Could you check a few things on this model? Use its own coordinates, in mm. Face numbers are marked on the shaded views. A direction names the side the tool comes from. Give positions to 0.01 mm unless a question says otherwise; leave off trailing zeros. Write each loop counter-clockwise with the first axis right and the second up, starting at its lowest first coordinate (ties: lowest second). Pieces come first, ordered by that corner, then holes. Notation, with made-up numbers: M 44.25,41.5 L 78.25,41.5 A15 ccw 78.25,68.5 Z; hole C 50.5,38 d11. An arc over 180 degrees is marked long. Use one line per item in the form item = value.
from build123d import *

# Parameters (mm, degrees)
SKETCH7_W           = 32.8
SKETCH7_H           = 24.5
BOSS_EXTRUDE3_DEPTH = 19
SKETCH8_W           = 29.8
SKETCH8_H           = 24.5
BOSS_EXTRUDE4_DEPTH = 7
CUT_EXTRUDE1_DEPTH  = 23.5
CUT_EXTRUDE2_REACH  = 44.494
SKETCH10_W          = 2.7
SKETCH10_H          = 21.05
SKETCH18_W          = 3
SKETCH18_H          = 8
CUT_EXTRUDE3_DEPTH  = 1
CHAMFER1_SIZE       = 0.5
CUT_EXTRUDE5_REACH  = 44.494
SKETCH20_R          = 0.6
CUT_EXTRUDE6_REACH  = 44.494
SKETCH19_R          = 0.6
CUT_EXTRUDE7_REACH  = 35.091
SKETCH21_R          = 2.25
SKETCH21_R_2        = 1.25
CHAMFER2_SIZE       = 0.5
CHAMFER4_SIZE       = 0.2


with BuildPart() as part:
    # Sketch7 → Boss-Extrude3 (new body)
    with BuildSketch(Plane.XY):
        Rectangle(SKETCH7_W, SKETCH7_H)
    extrude(amount=BOSS_EXTRUDE3_DEPTH)

    # Sketch8 → Boss-Extrude4 (add)
    with BuildSketch(Plane.XY.offset(19)):
        Rectangle(SKETCH8_W, SKETCH8_H)
    extrude(amount=BOSS_EXTRUDE4_DEPTH)

    # Sketch16 → Cut-Extrude1 (cut)
    with BuildSketch(Plane.XY.offset(26)):
        with BuildLine():
            Line((-12.4, -11.25), (12.4, -11.25))
            ThreePointArc((12.4, -11.25), (13.460660172, -10.810660172), (13.9, -9.75))
            Line((13.9, -9.75), (13.9, 9.75))
            ThreePointArc((13.9, 9.75), (13.460660172, 10.810660172), (12.4, 11.25))
            Line((12.4, 11.25), (-12.4, 11.25))
            ThreePointArc((-12.4, 11.25), (-13.460660172, 10.810660172), (-13.9, 9.75))
            Line((-13.9, 9.75), (-13.9, -9.75))
            ThreePointArc((-13.9, -9.75), (-13.460660172, -10.810660172), (-12.4, -11.25))
        make_face()
    extrude(amount=-CUT_EXTRUDE1_DEPTH, mode=Mode.SUBTRACT)

    # Cut-Extrude2: up to this face of the body (flat: up to its plane)
    cut_extrude2_end = Plane(part.part.faces().sort_by_distance((14.9, 0, 22.5))[0])
    # Sketch10 → Cut-Extrude2 (cut, up to the picked face)
    with BuildSketch(Plane.ZY.offset(14.9), mode=Mode.PRIVATE) as cut_extrude2_sk1:
        with Locations((24.65, 0.725)):
            Rectangle(SKETCH10_W, SKETCH10_H)
    cut_extrude2_tool1 = split(extrude(cut_extrude2_sk1.sketch, amount=-CUT_EXTRUDE2_REACH, mode=Mode.PRIVATE), bisect_by=cut_extrude2_end, keep=Keep.BOTH, mode=Mode.PRIVATE)
    add(cut_extrude2_tool1.solids().sort_by(Axis((-14.9, 0.725, 24.65), (1, 0, 0)))[0], mode=Mode.SUBTRACT)

    # Sketch18 → Cut-Extrude3 (cut)
    with BuildSketch(Plane(origin=(14.9, 0, 0), x_dir=(0, 0, -1), z_dir=(1, 0, 0))):
        with Locations((-21.8, 3.95)):
            Rectangle(SKETCH18_W, SKETCH18_H)
    extrude(amount=-CUT_EXTRUDE3_DEPTH, mode=Mode.SUBTRACT)

    # Chamfer1
    chamfer1_edges = [part.edges().sort_by_distance(p)[0] for p in [
        (0, -12.25, 0),
        (-16.4, 0, 0),
        (0, 12.25, 0),
        (16.4, 0, 0),
        (16.4, -12.25, 9.5),
        (-16.4, -12.25, 9.5),
        (-16.4, 12.25, 9.5),
        (16.4, 12.25, 9.5),
    ]]
    chamfer(chamfer1_edges, length=CHAMFER1_SIZE)

    # Sketch20 → Cut-Extrude5 (cut, up to next)
    with BuildSketch(Plane(origin=(14.9, 0, 0), x_dir=(0, 0, -1), z_dir=(1, 0, 0)), mode=Mode.PRIVATE) as cut_extrude5_sk1:
        with Locations((-21.5, 10)):
            Circle(SKETCH20_R)
    cut_extrude5_tool1 = extrude(cut_extrude5_sk1.sketch, amount=-CUT_EXTRUDE5_REACH, mode=Mode.PRIVATE) & part.part
    # Sketch20 → Cut-Extrude5 (cut, up to next)
    with BuildSketch(Plane(origin=(14.9, 0, 0), x_dir=(0, 0, -1), z_dir=(1, 0, 0)), mode=Mode.PRIVATE) as cut_extrude5_sk2:
        with Locations((-21.5, -10)):
            Circle(SKETCH20_R)
    cut_extrude5_tool2 = extrude(cut_extrude5_sk2.sketch, amount=-CUT_EXTRUDE5_REACH, mode=Mode.PRIVATE) & part.part
    add(cut_extrude5_tool1.solids().sort_by_distance((14.9, 10, 21.5))[0], mode=Mode.SUBTRACT)
    add(cut_extrude5_tool2.solids().sort_by_distance((14.9, -10, 21.5))[0], mode=Mode.SUBTRACT)

    # Sketch19 → Cut-Extrude6 (cut, up to next)
    with BuildSketch(Plane.ZY.offset(14.9), mode=Mode.PRIVATE) as cut_extrude6_sk1:
        with Locations(Location((21.5, 10, 0), (0, 0, 180))):
            Circle(SKETCH19_R)
    cut_extrude6_tool1 = extrude(cut_extrude6_sk1.sketch, amount=-CUT_EXTRUDE6_REACH, mode=Mode.PRIVATE) & part.part
    # Sketch19 → Cut-Extrude6 (cut, up to next)
    with BuildSketch(Plane.ZY.offset(14.9), mode=Mode.PRIVATE) as cut_extrude6_sk2:
        with Locations(Location((21.5, -10, 0), (0, 0, 180))):
            Circle(SKETCH19_R)
    cut_extrude6_tool2 = extrude(cut_extrude6_sk2.sketch, amount=-CUT_EXTRUDE6_REACH, mode=Mode.PRIVATE) & part.part
    add(cut_extrude6_tool1.solids().sort_by_distance((-14.9, 10, 21.5))[0], mode=Mode.SUBTRACT)
    add(cut_extrude6_tool2.solids().sort_by_distance((-14.9, -10, 21.5))[0], mode=Mode.SUBTRACT)

    # Sketch21 → Cut-Extrude7 (cut, up to next)
    with BuildSketch(Plane(origin=(0, 0, 0), x_dir=(-1, 0, 0), z_dir=(0, 0, -1)), mode=Mode.PRIVATE) as cut_extrude7_sk1:
        with Locations((-10.65, 0)):
            Circle(SKETCH21_R)
    cut_extrude7_tool1 = extrude(cut_extrude7_sk1.sketch, amount=-CUT_EXTRUDE7_REACH, mode=Mode.PRIVATE) & part.part
    # Sketch21 → Cut-Extrude7 (cut, up to next)
    with BuildSketch(Plane(origin=(0, 0, 0), x_dir=(-1, 0, 0), z_dir=(0, 0, -1)), mode=Mode.PRIVATE) as cut_extrude7_sk2:
        with Locations((0, 6)):
            Circle(SKETCH21_R_2)
    cut_extrude7_tool2 = extrude(cut_extrude7_sk2.sketch, amount=-CUT_EXTRUDE7_REACH, mode=Mode.PRIVATE) & part.part
    # Sketch21 → Cut-Extrude7 (cut, up to next)
    with BuildSketch(Plane(origin=(0, 0, 0), x_dir=(-1, 0, 0), z_dir=(0, 0, -1)), mode=Mode.PRIVATE) as cut_extrude7_sk3:
        with Locations((0, -6)):
            Circle(SKETCH21_R_2)
    cut_extrude7_tool3 = extrude(cut_extrude7_sk3.sketch, amount=-CUT_EXTRUDE7_REACH, mode=Mode.PRIVATE) & part.part
    add(cut_extrude7_tool1.solids().sort_by_distance((10.65, 0, 0))[0], mode=Mode.SUBTRACT)
    add(cut_extrude7_tool2.solids().sort_by_distance((0, 6, 0))[0], mode=Mode.SUBTRACT)
    add(cut_extrude7_tool3.solids().sort_by_distance((0, -6, 0))[0], mode=Mode.SUBTRACT)

    # Chamfer2
    chamfer2_edges = [part.edges().sort_by_distance(p)[0] for p in [
        (12.9, 0, 0),
    ]]
    chamfer(chamfer2_edges, length=CHAMFER2_SIZE)

    # Chamfer4
    chamfer4_edges = [part.edges().sort_by_distance(p)[0] for p in [
        (1.25, 6, 2.5),
        (1.25, 6, 0),
        (1.25, -6, 2.5),
        (1.25, -6, 0),
        (12.9, 0, 2.5),
    ]]
    chamfer(chamfer4_edges, length=CHAMFER4_SIZE)


solid = part.part
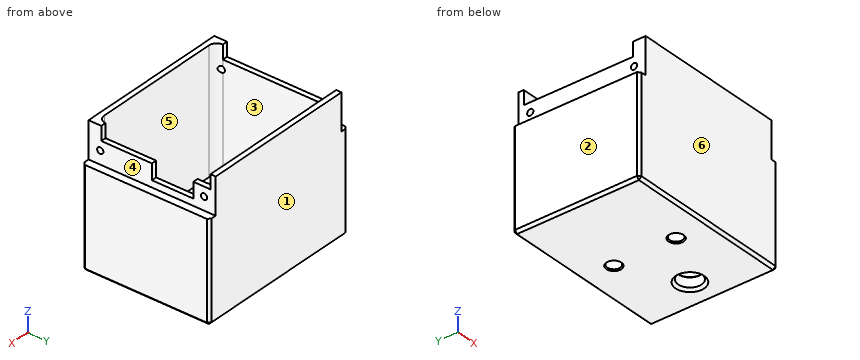
1) Thinking about a two-plate mould opening in Y: for the marked faces 1, 2 and 3, which applies, released by +Y, released by -Y, zero draft, split by the parting line, or undercut?
Checked values:
face_1 = released by +Y
face_2 = zero draft
face_3 = undercut
2) I want a section at B-B, the plane y = 6. Please give me the cut outline in (x, z), plus the area to 3 significant figures.
Checked values:
outline = M -16.4,0.5 L -15.9,0 L -1.45,0 L -1.25,0.2 L -1.25,2.3 L -1.45,2.5 L -13.9,2.5 L -13.9,23.3 L -14.9,23.3 L -14.9,19 L -16.4,19 Z; M 1.25,0.2 L 1.45,0 L 15.9,0 L 16.4,0.5 L 16.4,19 L 14.9,19 L 14.9,20.3 L 13.9,20.3 L 13.9,2.5 L 1.45,2.5 L 1.25,2.3 Z
area = 164 mm2
3) For pin 1 Ø1.1 at (x, y) = (14, -7.5) entering from +Z; pin 2 Ø2 at (y, z) = (-4.5, 22.5) entering from -X; pin 3 Ø1 at (x, y) = (0, 3) entering from -Z; pin 4 Ø3 at (x, y) = (11.5, 5) entering from +Z, each with a flat end and sliding along its axis, tell me the tip position at first contact or that it passes through.
Checked values:
pin_1 = 23.3
pin_2 = -14.9
pin_3 = 0
pin_4 = 2.5
4) If I drill on L1, parallel to Y at x = 0, z = 1.2; L2, parallel to Y at x = 11, z = 4.25; L3, parallel to Z at x = 14.4, y = -10, over which ranges is the centre line in solid material (lowest first)?
Checked values:
L1 = -12.25 to -7.25, -4.75 to 4.75, 7.25 to 12.25
L2 = -12.25 to -11.25, 11.25 to 12.25
L3 = 0 to 20.9, 22.1 to 26
5) I want a section at C-C, the plane z = 3. Please give me the cut outline in (x, y).
Checked values:
outline = M -16.4,-11.75 L -15.9,-12.25 L 15.9,-12.25 L 16.4,-11.75 L 16.4,11.75 L 15.9,12.25 L -15.9,12.25 L -16.4,11.75 Z; hole M -13.9,-9.75 A1.5 ccw -12.4,-11.25 L 12.4,-11.25 A1.5 ccw 13.9,-9.75 L 13.9,9.75 A1.5 ccw 12.4,11.25 L -12.4,11.25 A1.5 ccw -13.9,9.75 Z
6) I want a section at A-A, the plane x = 0. Please give me the cut outline in (y, z).
Checked values:
outline = M -12.25,0.5 L -11.75,0 L -7.45,0 L -7.25,0.2 L -7.25,2.3 L -7.45,2.5 L -11.25,2.5 L -11.25,26 L -12.25,26 Z; M -4.75,0.2 L -4.55,0 L 4.55,0 L 4.75,0.2 L 4.75,2.3 L 4.55,2.5 L -4.55,2.5 L -4.75,2.3 Z; M 7.25,0.2 L 7.45,0 L 11.75,0 L 12.25,0.5 L 12.25,26 L 11.25,26 L 11.25,2.5 L 7.45,2.5 L 7.25,2.3 Z
7) For the marked faces 4, 5 and 6, which set-ups out of +Z, -Z, +X, -X, +Y, -Y let a thin tool reach every point of the face, with its end or its side?
Checked values:
face_4 = +Z, +X, +Y, -Y
face_5 = +Z
face_6 = +Z, -Z, +X, -X, -Y
8) I want a section at D-D, the plane y = -3.5. Please give me the cut outline in (x, z).
Checked values:
outline = M -16.4,0.5 L -15.9,0 L 15.9,0 L 16.4,0.5 L 16.4,19 L 14.9,19 L 14.9,23.3 L 13.9,23.3 L 13.9,2.5 L -13.9,2.5 L -13.9,23.3 L -14.9,23.3 L -14.9,19 L -16.4,19 Z
